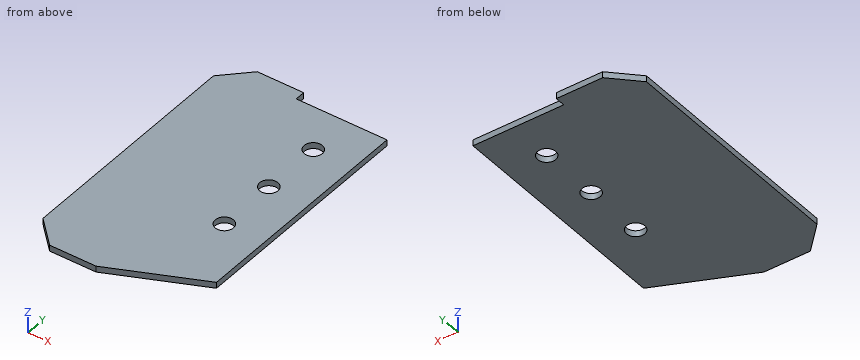
Autodesk Fusion 360 part; units mm, degrees
sketch "スケッチ1" plane through (0, 0, 0) normal (0, 0, 1) x (1, 0, 0)
  line L0 (-9.5, 140) -> (-80.5, 140)
  line L1 (-80.5, 140) -> (-80.5, -140)
  line L2 (-80.5, -140) -> (-9.5, -140)
  line L3 (80.5, -100) -> (80.5, 130)
  line L4 (74.75, 130) -> (-80.5, -140) construction
  line L5 (-80.5, 140) -> (62.1814, -108.1416) construction
  line L6 (-9.5, 140) -> (-9.5, 130)
  line L7 (-9.5, 130) -> (80.5, 130)
  line L8 (-80.5, -140) -> (-9.5, -140) construction
  line L9 (80.5, -100) -> (-9.5, -140)
  dimension "d2" = 280
  dimension "d5" = 71
extrude "押し出し1" add sketch "スケッチ1" along normal blind 6
chamfer "面取り1" distance 25 angle 45 2 edges at (-80.5, -140, 3) (-80.5, 140, 3)
sketch "スケッチ2" plane through (0, 0, 6) normal (0, 0, 1) x (-1, 0, 0)
  line L0 (55.5, -140) -> (80.5, -115)
  line L1 (80.5, -115) -> (80.5, 115)
  line L2 (80.5, 115) -> (55.5, 140)
  line L3 (55.5, 140) -> (9.5, 140)
  line L4 (9.5, 140) -> (-80.5, 100)
  line L5 (-80.5, 100) -> (-80.5, -130)
  line L6 (-80.5, -130) -> (9.5, -130)
  line L7 (9.5, -130) -> (9.5, -140)
  line L8 (9.5, -140) -> (55.5, -140)
  line L9 (-80.5, -130) -> (-40.5, -130) construction
  line L10 (-40.5, -130) -> (-40.5, -85) construction
  line L11 (-40.5, -85) -> (-80.5, -85) construction
  line L12 (-80.5, -85) -> (-80.5, -130) construction
  line L13 (-40.5, -85) -> (-40.5, -25) construction
  line L14 (-40.5, -25) -> (-40.5, 35) construction
  point P0 (-40.5, -85)
  point P1 (-40.5, -25)
  point P2 (-40.5, 35)
  dimension "d10" = 40
  dimension "d11" = 45
  dimension "d12" = 60
  dimension "d13" = 60
hole "穴1" at (40.5, 85, 6) at (40.5, 25, 6) at (40.5, -35, 6) direction (0, 0, -1) diameter 18 end through all
equation "d5 = 25 mm + 46 mm"
Input: part model. Units: mm. Frame: model coordinates. Coordinates: 2 decimals unless noted, no trailing zeros. Loops run counter-clockwise (first coordinate to the right, second up) from the corner with the lowest first, then second, coordinate; pieces in that order, holes last. Notation, with made-up numbers: M 55.25,-25 L 100.25,-25 A24 ccw 100.25,8 Z; hole C 24.25,61.25 d7. An arc over 180 degrees is marked long. Use a Markdown table: item, result. Add a question column.
1) Pin query (flat end, axial travel): P1, Ø3, axis at y = 133.5, z = 3, coming from the +X side; P2, Ø1, axis at x = -2.5, z = 5.5, coming from the +Y side. Return the tip coordinate at first contact, or that it passes through.
2) Section B-B, the plane z = 3.65. Return the cut outline in (x, y).
3) Section C-C, the plane x = 46. Return the cut outline in (y, z), plus the area to 3 significant figures.
4) Line query: L1, parallel to X at y = -35, z = 1.3; L2, parallel to Y at x = 40.5, z = 2.8; L3, parallel to Y at x = 45.5, z = 1.15. Output: solid intervals per line, ascending. Write a range as from..to.
5) Section A-A, the plane y = 85. Return the cut outline in (x, z).
6) Section D-D, the plane y = -41. Return the cut outline in (x, z).
Answer below:
| question | item | result |
|---|---|---|
| 1 | P1 | x = -9.5 |
| 1 | P2 | y = 130 |
| 2 | outline | M -80.5,-115 L -55.5,-140 L -9.5,-140 L 80.5,-100 L 80.5,130 L -9.5,130 L -9.5,140 L -55.5,140 L -80.5,115 Z; hole C 40.5,-35 d18; hole C 40.5,25 d18; hole C 40.5,85 d18 |
| 3 | outline | M -115.33,0 L -42.12,0 L -42.12,6 L -115.33,6 Z; M -27.88,0 L 17.88,0 L 17.88,6 L -27.88,6 Z; M 32.12,0 L 77.88,0 L 77.88,6 L 32.12,6 Z; M 92.12,0 L 130,0 L 130,6 L 92.12,6 Z |
| 3 | area | 1,220 mm2 |
| 4 | L1 | -80.5..31.5, 49.5..80.5 |
| 4 | L2 | -117.78..-44, -26..16, 34..76, 94..130 |
| 4 | L3 | -115.56..-42.48, -27.52..17.52, 32.48..77.52, 92.48..130 |
| 5 | outline | M -80.5,0 L 31.5,0 L 31.5,6 L -80.5,6 Z; M 49.5,0 L 80.5,0 L 80.5,6 L 49.5,6 Z |
| 6 | outline | M -80.5,0 L 33.79,0 L 33.79,6 L -80.5,6 Z; M 47.21,0 L 80.5,0 L 80.5,6 L 47.21,6 Z |
